Study the drawing (mm; zero at the part's minimum x, y, z) and answer. Coordinates: 2 decimals unless noted, no trailing zeros. Write each loop counter-clockwise with the first axis right and the second up, starting at its lowest first coordinate (ties: lowest second). Pieces come first, ordered by that corner, then holes. Notation, with made-up numbers: (6.5, -39) - (56.5, -39) arc R19 ccw to (56.5, -16) - close; hole circle Ø4 at (19, 30). An arc over 180 degrees is marked (long way). One line per item, written item: value.
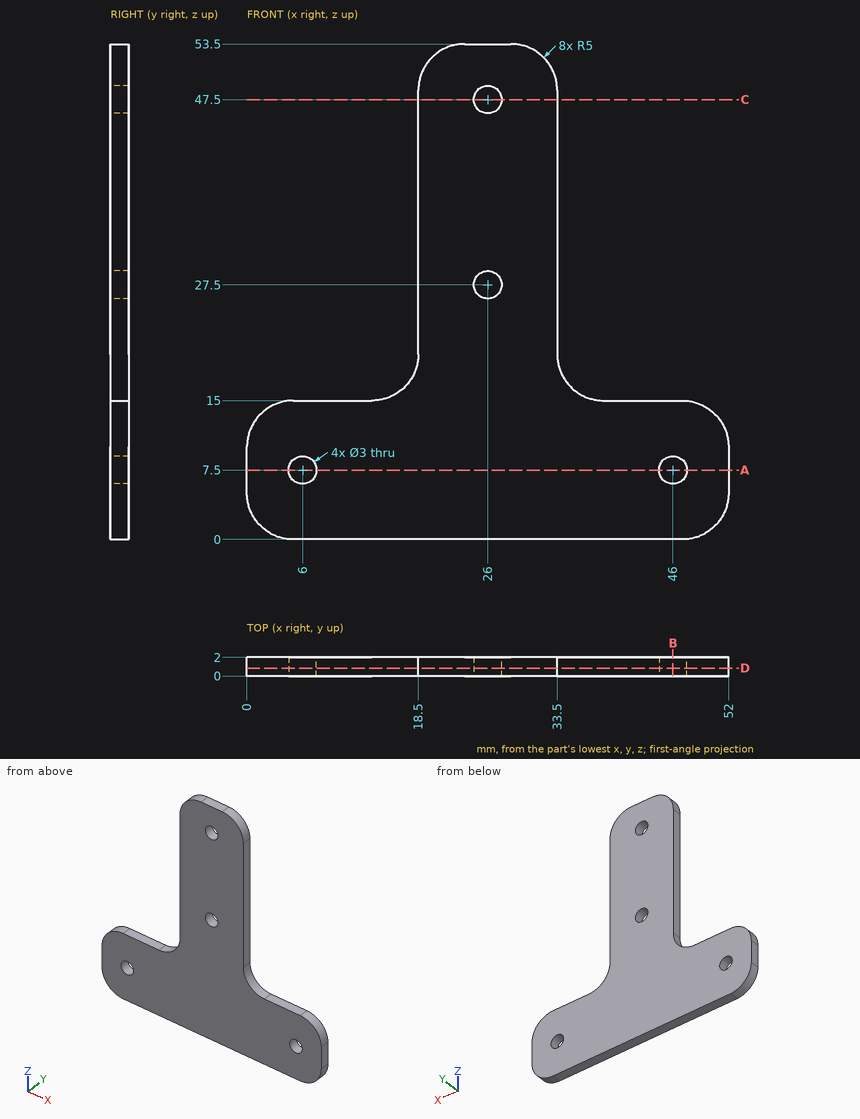
Item 1: Section D-D, the plane y = 0.85 is taken. Determine the outline of the cut face in (x, z).
Evaluation:
outline: (0, 5) arc R5 ccw to (5, 0) - (47, 0) arc R5 ccw to (52, 5) - (52, 10) arc R5 ccw to (47, 15) - (38.5, 15) arc R5 cw to (33.5, 20) - (33.5, 48.5) arc R5 ccw to (28.5, 53.5) - (23.5, 53.5) arc R5 ccw to (18.5, 48.5) - (18.5, 20) arc R5 cw to (13.5, 15) - (5, 15) arc R5 ccw to (0, 10) - close; hole circle Ø3 at (6, 7.5); hole circle Ø3 at (26, 27.5); hole circle Ø3 at (26, 47.5); hole circle Ø3 at (46, 7.5)
Item 2: Consider probe 1 along X at (y, z) = (0.6, 47.5); probe 2 along Z at (x, y) = (26, 1.1); probe 3 along X at (y, z) = (1.25, 21). Determine where each line is inside the solid, lowest interval first.
Evaluation:
probe 1: x = 18.5 to 24.5, 27.5 to 33.5
probe 2: z = 0 to 26, 29 to 46, 49 to 53.5
probe 3: x = 18.5 to 33.5
Item 3: Section C-C, the plane z = 47.5 is taken. Determine the outline of the cut face in (x, y).
Evaluation:
outline: (18.5, 0) - (24.5, 0) - (24.5, 2) - (18.5, 2) - close; (27.5, 0) - (33.5, 0) - (33.5, 2) - (27.5, 2) - close
Item 4: Given pin 1 (2.5 mm diameter, centred on x = 26, z = 27.5, fed in from -Y); pin 2 (5 mm diameter, centred on x = 35.5, z = 34, fed in from -Y), each flat-ended and moving along its own axis, determine where each tip first touches the part or whether it passes through.
Evaluation:
pin 1: passes through
pin 2: stops at y = 0
Item 5: Section A-A, the plane z = 7.5 is taken. Determine the outline of the cut face in (x, y), then the cut area to 3 significant figures.
Evaluation:
outline: (0, 0) - (4.5, 0) - (4.5, 2) - (0, 2) - close; (7.5, 0) - (44.5, 0) - (44.5, 2) - (7.5, 2) - close; (47.5, 0) - (52, 0) - (52, 2) - (47.5, 2) - close
area: 92.0 mm2
Item 6: Section B-B, the plane x = 46 is taken. Determine the outline of the cut face in (y, z).
Evaluation:
outline: (0, 0) - (2, 0) - (2, 6) - (0, 6) - close; (0, 9) - (2, 9) - (2, 15) - (0, 15) - close
